```python
from build123d import *

# Parameters (mm, degrees)
SKETCH_1_W          = 20
SKETCH_1_H          = 10
SKETCH_1_W_2        = 16
SKETCH_1_H_2        = 6
EXTRUDE_1_DEPTH     = 125
SKETCH_3_R          = 2.05
CUT_EXTRUDE_1_DEPTH = 126.800383248


with BuildPart() as part:
    # 草图1 → 凸台-拉伸1 (new, symmetric)
    with BuildSketch(Plane.XY):
        with Locations((0.036753729, 0.03823935)):
            Rectangle(SKETCH_1_W, SKETCH_1_H)
        with Locations((0.036753729, 0.03823935)):
            Rectangle(SKETCH_1_W_2, SKETCH_1_H_2, mode=Mode.SUBTRACT)
    extrude(amount=EXTRUDE_1_DEPTH, both=True)

    # 草图3 → 切除-拉伸1 (cut, through all)
    with BuildSketch(Plane(origin=(0, 5.03823935, 0), x_dir=(1, 0, 0), z_dir=(0, 1, 0))):
        with Locations(Location((-4.963246271, 110, 0), (0, 0, 270))):
            Circle(SKETCH_3_R)
        with Locations(Location((5.036753729, 110, 0), (0, 0, 270))):
            Circle(SKETCH_3_R)
    cut_extrude_1 = extrude(amount=-CUT_EXTRUDE_1_DEPTH, mode=Mode.SUBTRACT)

    # 镜向1: 切除-拉伸1 across plane
    add(cut_extrude_1.mirror(Plane.XY), mode=Mode.SUBTRACT)


solid = part.part
```
Geometry check sheet. Reference: the model listing, model coordinates, mm. A direction names the side the tool comes from. Give positions to 0.01 mm unless a question says otherwise; leave off trailing zeros. Loops run counter-clockwise (first coordinate to the right, second up) from the corner with the lowest first, then second, coordinate; pieces in that order, holes last. Notation, with made-up numbers: (-25, 40) - (33, 40) arc R6 ccw to (33, 44) - close; hole circle Ø3 at (85, 52). An arc over 180 degrees is marked (long way). Use CSV: the item, a comma, the result in double quotes. Start each with the question number.
Q1. Access from +Z, -Z, +X, -X, +Y, -Y to the whole of each face (thin tool, end or side, straight path). Record for faces 5 (the face through (8.037, 0, 2)), 6 (the face through (10.037, 0, 2)).
Q2. Go/stop test with flat-tipped pins: pin 1 Ø3.5 at (x, z) = (5.04, 110) entering from -Y; pin 2 Ø6.5 at (x, z) = (5.04, -110) entering from -Y. Record where each tip stops, or that it passes through.
Q3. Section check C-C, the plane z = -25. Record the cut outline in (x, y).
Q4. Section check A-A, the plane z = -110. Record the cut outline in (x, y).
Q5. Release check for a two-part mould opening along Y. For faces 1 (the face through (0, -2.962, 2)), 2 (the face through (0, 3.038, 2)), 3 (the face through (0, 5.038, 2)), 4 (the face through (-4.347, 4.052, 108.045)) record: +Y half, -Y half, draft (parallel to the pull), parting line (faces both ways), or undercut.
Q6. Scan lines: probe 1 along X at (y, z) = (-4, 110); probe 2 along X at (y, z) = (-1.5, -78.5); probe 3 along Y at (x, z) = (-6, -6.5). Record each from-to range of solid material in increasing order. Write a range as from..to.
Q7. Section check B-B, the plane y = 0.5. Record the cut outline in (x, z).
Findings below:
1,face 5,"+Z, -Z"
1,face 6,"+Z, -Z, +X, +Y, -Y"
2,pin 1,"passes through"
2,pin 2,"stops at y = -4.96"
3,outline,"(-9.96, -4.96) - (10.04, -4.96) - (10.04, 5.04) - (-9.96, 5.04) - close; hole (-7.96, -2.96) - (8.04, -2.96) - (8.04, 3.04) - (-7.96, 3.04) - close"
4,outline,"(-9.96, -4.96) - (-7.01, -4.96) - (-7.01, -2.96) - (-7.96, -2.96) - (-7.96, 3.04) - (-7.01, 3.04) - (-7.01, 5.04) - (-9.96, 5.04) - close; (-2.91, -4.96) - (2.99, -4.96) - (2.99, -2.96) - (-2.91, -2.96) - close; (-2.91, 3.04) - (2.99, 3.04) - (2.99, 5.04) - (-2.91, 5.04) - close; (7.09, -4.96) - (10.04, -4.96) - (10.04, 5.04) - (7.09, 5.04) - (7.09, 3.04) - (8.04, 3.04) - (8.04, -2.96) - (7.09, -2.96) - close"
5,face 1,"undercut"
5,face 2,"undercut"
5,face 3,"+Y half"
5,face 4,"draft"
6,probe 1,"x = -9.96..-7.01, -2.91..2.99, 7.09..10.04"
6,probe 2,"x = -9.96..-7.96, 8.04..10.04"
6,probe 3,"y = -4.96..-2.96, 3.04..5.04"
7,outline,"(-9.96, -125) - (-7.96, -125) - (-7.96, 125) - (-9.96, 125) - close; (8.04, -125) - (10.04, -125) - (10.04, 125) - (8.04, 125) - close"
